from build123d import *

# Parameters (mm, degrees)
SKETCH1_W           = 50
SKETCH1_H           = 38
SKETCH1_R           = 2.4
SKETCH1_W_2         = 23.5
SKETCH1_H_2         = 12
BOSS_EXTRUDE1_DEPTH = 4
CUT_EXTRUDE1_REACH  = 6
SKETCH2_R           = 1


with BuildPart() as part:
    # Sketch1 → Boss-Extrude1 (new body)
    with BuildSketch(Plane.XY):
        with Locations((0, -19)):
            Rectangle(SKETCH1_W, SKETCH1_H)
        with Locations((-19.92, -7.045)):
            Circle(SKETCH1_R, mode=Mode.SUBTRACT)
        with Locations((-19.92, -30.955)):
            Circle(SKETCH1_R, mode=Mode.SUBTRACT)
        with Locations((19.92, -30.955)):
            Circle(SKETCH1_R, mode=Mode.SUBTRACT)
        with Locations((19.92, -7.045)):
            Circle(SKETCH1_R, mode=Mode.SUBTRACT)
        with Locations((0, -19)):
            Rectangle(SKETCH1_W_2, SKETCH1_H_2, mode=Mode.SUBTRACT)
    extrude(amount=BOSS_EXTRUDE1_DEPTH)

    # Sketch2 → Cut-Extrude1 (cut, up to next)
    with BuildSketch(Plane.XY.offset(4), mode=Mode.PRIVATE) as cut_extrude1_sk1:
        with Locations((-14.5, -19)):
            Circle(SKETCH2_R)
    cut_extrude1_tool1 = extrude(cut_extrude1_sk1.sketch, amount=-CUT_EXTRUDE1_REACH, mode=Mode.PRIVATE) & part.part
    add(cut_extrude1_tool1.solids().sort_by_distance((-14.5, -19, 4))[0], mode=Mode.SUBTRACT)
    # Sketch2 → Cut-Extrude1 (cut, up to next)
    with BuildSketch(Plane.XY.offset(4), mode=Mode.PRIVATE) as cut_extrude1_sk2:
        with Locations((14.5, -19)):
            Circle(SKETCH2_R)
    cut_extrude1_tool2 = extrude(cut_extrude1_sk2.sketch, amount=-CUT_EXTRUDE1_REACH, mode=Mode.PRIVATE) & part.part
    add(cut_extrude1_tool2.solids().sort_by_distance((14.5, -19, 4))[0], mode=Mode.SUBTRACT)


solid = part.part
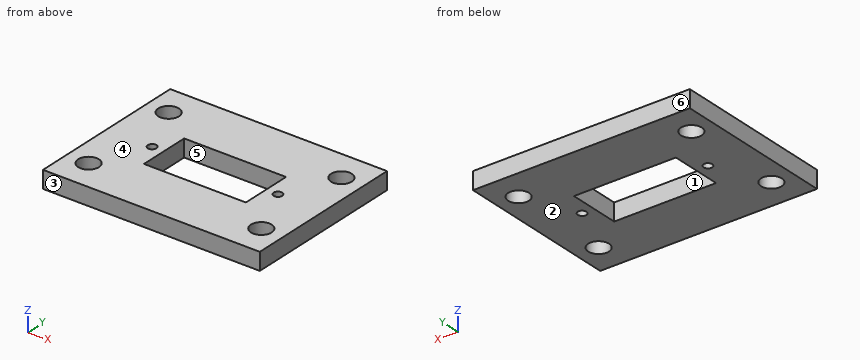
Read the model definition and answer for the solid it produces. Units are mm, in the model's axes. Face numbers are marked on the shaded views. A direction names the side the tool comes from. Round coordinates to 2 decimals unless told otherwise and drop trailing zeros. Loops run counter-clockwise (first coordinate to the right, second up) from the corner with the lowest first, then second, coordinate; pieces in that order, holes last. Notation, with made-up numbers: (26.5, -16.75) - (51.5, -16.75) arc R22 ccw to (51.5, 22.25) - close; hole circle Ø3 at (77.5, 24). An arc over 180 degrees is marked (long way). One line per question, with ' | ' between items. Start each with the question number.
Q1. For a pull along Y with two mould halves and no side action, classify the marked faces 3, 4, 5 and 6 as +Y half, -Y half, draft (parallel to the pull), parting line (faces both ways), or undercut.
Q2. Section C-C on x = 19.92 is taken. Give the vertices of the cut face in (y, z) (3 decimals), plus the area to 3 significant figures.
Q3. For the marked faces 1 and 2, determine the directions among +Z, -Z, +X, -X, +Y, -Y from which every point of the face is accessible in a straight line to the end or side of a thin tool.
Q4. Section B-B on y = -14.5 is taken. Give the vertices of the cut face in (x, z), plus the area to 3 significant figures.
Q5. Section A-A on x = 14.5 is taken. Give the vertices of the cut face in (y, z).
Q6. Find the intervals of material crossed by L1, parallel to Y at x = -20, z = 1.1; L2, parallel to X at y = -31, z = 0.35; L3, parallel to X at y = -21.5, z = 2.5, in increasing order.
Q7. A flat-ended cylindrical pin translates along its axis: pin 1 (1.2 mm diameter, centred on x = 14.5, y = -19, fed in from -Z). Find the tip coordinate at first contact, or state that the pin passes through.
Q8. Section D-D on z = 3.4 is taken. Give the vertices of the cut face in (x, y) (3 decimals), plus the area to 3 significant figures.
Established:
1) face 3: -Y half | face 4: draft | face 5: undercut | face 6: +Y half
2) outline: (-38, 0) - (-33.355, 0) - (-33.355, 4) - (-38, 4) - close; (-28.555, 0) - (-9.445, 0) - (-9.445, 4) - (-28.555, 4) - close; (-4.645, 0) - (0, 0) - (0, 4) - (-4.645, 4) - close | area: 114 mm²
3) face 1: +Z, -Z | face 2: -Z, +X, -X, +Y, -Y
4) outline: (-25, 0) - (-11.75, 0) - (-11.75, 4) - (-25, 4) - close; (11.75, 0) - (25, 0) - (25, 4) - (11.75, 4) - close | area: 106 mm²
5) outline: (-38, 0) - (-20, 0) - (-20, 4) - (-38, 4) - close; (-18, 0) - (0, 0) - (0, 4) - (-18, 4) - close
6) L1: -38 to -33.35, -28.56 to -9.44, -4.65 to 0 | L2: -25 to -22.32, -17.52 to 17.52, 22.32 to 25 | L3: -25 to -11.75, 11.75 to 25
7) pin 1: through
8) outline: (-25, -38) - (25, -38) - (25, 0) - (-25, 0) - close; hole circle Ø4.8 at (-19.92, -30.955); hole circle Ø4.8 at (-19.92, -7.045); hole circle Ø2 at (-14.5, -19); hole (-11.75, -25) - (11.75, -25) - (11.75, -13) - (-11.75, -13) - close; hole circle Ø2 at (14.5, -19); hole circle Ø4.8 at (19.92, -30.955); hole circle Ø4.8 at (19.92, -7.045) | area: 1,540 mm²
